from build123d import *

# Parameters (mm, degrees)
SKIZZE1_W                       = 22
SKIZZE1_H                       = 72.8
AUFSATZ_LINEAR_AUSTRAGEN1_DEPTH = 2
SKIZZE2_R                       = 3
SCHNITT_LINEAR_AUSTRAGEN1_DEPTH = 2
SKIZZE3_W                       = 65.5
SKIZZE3_H                       = 21
AUFSATZ_LINEAR_AUSTRAGEN2_DEPTH = 2.8
SCHNITT_LINEAR_AUSTRAGEN2_DEPTH = 67.590464783
SKIZZE5_R                       = 3
SCHNITT_LINEAR_AUSTRAGEN4_DEPTH = 39.128729326
SKIZZE6_W                       = 18
SKIZZE6_H                       = 1
SCHNITT_LINEAR_AUSTRAGEN5_DEPTH = 40
SKIZZE8_W                       = 15
SKIZZE8_H                       = 10
SCHNITT_LINEAR_AUSTRAGEN6_DEPTH = 0.5
VERRUNDUNG3_R                   = 1
SKIZZE9_W                       = 5
SKIZZE9_H                       = 12
AUFSATZ_LINEAR_AUSTRAGEN3_DEPTH = 8
SKIZZE10_W                      = 10
SKIZZE10_H                      = 5
SCHNITT_LINEAR_AUSTRAGEN7_DEPTH = 75.236715983


with BuildPart() as part:
    # Skizze1 → Aufsatz-Linear austragen1 (new body)
    with BuildSketch(Plane(origin=(0, 0, 0), x_dir=(0, 1, 0), z_dir=(0, 0, 1))):
        Rectangle(SKIZZE1_W, SKIZZE1_H)
    extrude(amount=AUFSATZ_LINEAR_AUSTRAGEN1_DEPTH)

    # Skizze2 → Schnitt-Linear austragen1 (cut)
    with BuildSketch(Plane.XY.offset(2)):
        with Locations((-34.28, 8.88)):
            Circle(SKIZZE2_R)
        with Locations((-34.28, -8.88)):
            Circle(SKIZZE2_R)
        with Locations((34.28, -8.88)):
            Circle(SKIZZE2_R)
        with Locations((34.28, 8.88)):
            Circle(SKIZZE2_R)
    extrude(amount=-SCHNITT_LINEAR_AUSTRAGEN1_DEPTH, mode=Mode.SUBTRACT)

    # Skizze3 → Aufsatz-Linear austragen2 (add)
    with BuildSketch(Plane.XY.offset(2)):
        with Locations((3.65, 0)):
            Rectangle(SKIZZE3_W, SKIZZE3_H)
    extrude(amount=AUFSATZ_LINEAR_AUSTRAGEN2_DEPTH)

    # Skizze4 → Schnitt-Linear austragen2 (cut, through all)
    with BuildSketch(Plane(origin=(-29.1, 0, 0), x_dir=(0, -1, 0), z_dir=(-1, 0, 0))):
        Polygon((-8, 4.8), (8, 4.8), (8, 4.1), (9, 4.1), (9, 2), (-9, 2), (-9, 4.1), (-8, 4.1), align=None)
    extrude(amount=-SCHNITT_LINEAR_AUSTRAGEN2_DEPTH, mode=Mode.SUBTRACT)

    # Skizze5 → Schnitt-Linear austragen4 (cut, through all)
    with BuildSketch(Plane(origin=(0, 0, 2), x_dir=(1, 0, 0), z_dir=(0, 0, -1))):
        with Locations((34.28, -8.88)):
            Circle(SKIZZE5_R)
        with Locations((34.28, 8.88)):
            Circle(SKIZZE5_R)
    extrude(amount=-SCHNITT_LINEAR_AUSTRAGEN4_DEPTH, mode=Mode.SUBTRACT)

    # Skizze6 → Schnitt-Linear austragen5 (cut)
    with BuildSketch(Plane(origin=(-36.4, 0, 0), x_dir=(0, -1, 0), z_dir=(-1, 0, 0))):
        with Locations((0, 2)):
            Rectangle(SKIZZE6_W, SKIZZE6_H)
    extrude(amount=-SCHNITT_LINEAR_AUSTRAGEN5_DEPTH, mode=Mode.SUBTRACT)

    # Skizze8 → Schnitt-Linear austragen6 (cut)
    with BuildSketch(Plane.XY.offset(2)):
        with Locations((8.655984658, -0.007335612)):
            Rectangle(SKIZZE8_W, SKIZZE8_H)
    extrude(amount=-SCHNITT_LINEAR_AUSTRAGEN6_DEPTH, mode=Mode.SUBTRACT)

    # Verrundung3
    # the kernel refuses this fillet: 1 mm, written as the material it adds along each edge
    with BuildSketch(Plane(origin=(3.6, -9, 1.5), x_dir=(0, 0, 1), z_dir=(0, 1, 0))) as verrundung3_piece_1:
        with BuildLine():
            CenterArc((1, -0.866025404), VERRUNDUNG3_R, 120, 60)
            Line((0, -0.866025404), (-0.02, -0.866025404))
            Line((-0.02, -0.866025404), (-0.02, 0))
            Line((-0.02, 0), (0, 0.02))
            ThreePointArc((0, 0.02), (0.25, 0.02), (0.49, 0.017320508))
            Line((0.49, 0.017320508), (0.5, 0))
        make_face()
    extrude(amount=3.992664388)
    with BuildSketch(Plane(origin=(3.6, -5.007335612, 1.5), x_dir=(0, 0, 1), z_dir=(1, 0, 0)), Plane(origin=(16.155984658, 4.992664388, 1.5), x_dir=(0, 0, 1), z_dir=(-1, 0, 0))) as verrundung3_piece_2:
        with BuildLine():
            CenterArc((1, -0.866025404), VERRUNDUNG3_R, 120, 60)
            Line((0, -0.866025404), (-0.02, -0.866025404))
            Line((-0.02, -0.866025404), (-0.02, 0))
            Line((-0.02, 0), (0, 0.02))
            ThreePointArc((0, 0.02), (0.25, 0.02), (0.49, 0.017320508))
            Line((0.49, 0.017320508), (0.5, 0))
        make_face()
    extrude(amount=12.555984658)
    with BuildSketch(Plane(origin=(3.6, 4.992664388, 1.5), x_dir=(0, 0, 1), z_dir=(0, 1, 0))) as verrundung3_piece_3:
        with BuildLine():
            CenterArc((1, -0.866025404), VERRUNDUNG3_R, 120, 60)
            Line((0, -0.866025404), (-0.02, -0.866025404))
            Line((-0.02, -0.866025404), (-0.02, 0))
            Line((-0.02, 0), (0, 0.02))
            ThreePointArc((0, 0.02), (0.25, 0.02), (0.49, 0.017320508))
            Line((0.49, 0.017320508), (0.5, 0))
        make_face()
    extrude(amount=4.007335612)
    with BuildSketch(Plane(origin=(16.155984658, -5.007335612, 1.5), x_dir=(0, 0, 1), z_dir=(0, 1, 0))) as verrundung3_piece_4:
        with BuildLine():
            CenterArc((1, -0.866025404), VERRUNDUNG3_R, 120, 60)
            Line((0, -0.866025404), (-0.02, -0.866025404))
            Line((-0.02, -0.866025404), (-0.02, 0))
            Line((-0.02, 0), (0, 0.02))
            ThreePointArc((0, 0.02), (0.25, 0.02), (0.49, 0.017320508))
            Line((0.49, 0.017320508), (0.5, 0))
        make_face()
    extrude(amount=10)
    with BuildSketch(Plane(origin=(3.6, -9, 1.5), x_dir=(0, 0, 1), z_dir=(0, 1, 0))) as verrundung3_piece_5a_section:
        with BuildLine():
            CenterArc((1, -0.866025404), VERRUNDUNG3_R, 120, 60)
            Line((0, -0.866025404), (-0.02, -0.866025404))
            Line((-0.02, -0.866025404), (-0.02, 0))
            Line((-0.02, 0), (0, 0.02))
            ThreePointArc((0, 0.02), (0.25, 0.02), (0.49, 0.017320508))
            Line((0.49, 0.017320508), (0.5, 0))
        make_face()
    verrundung3_piece_5a = extrude(amount=6.157727897, mode=Mode.PRIVATE)
    verrundung3_piece_5a = split(verrundung3_piece_5a, bisect_by=Plane(origin=(3.383689554, -5.007335612, 1.629516711), z_dir=(0, 1, 0)), keep=Keep.TOP, mode=Mode.PRIVATE)
    with BuildSketch(Plane(origin=(1.434936491, -5.007335612, 1.5), x_dir=(0, 0, 1), z_dir=(1, 0, 0))) as verrundung3_piece_5b_section:
        with BuildLine():
            CenterArc((1, -0.866025404), VERRUNDUNG3_R, 120, 60)
            Line((0, -0.866025404), (-0.02, -0.866025404))
            Line((-0.02, -0.866025404), (-0.02, 0))
            Line((-0.02, 0), (0, 0.02))
            ThreePointArc((0, 0.02), (0.25, 0.02), (0.49, 0.017320508))
            Line((0.49, 0.017320508), (0.5, 0))
        make_face()
    verrundung3_piece_5b = extrude(amount=14.721048168, mode=Mode.PRIVATE)
    verrundung3_piece_5b = split(verrundung3_piece_5b, bisect_by=Plane(origin=(3.6, -4.791025166, 1.629516711), z_dir=(-1, 0, 0)), keep=Keep.TOP, mode=Mode.PRIVATE)
    verrundung3_piece_5 = verrundung3_piece_5a & verrundung3_piece_5b
    add(verrundung3_piece_5)
    with BuildSketch(Plane(origin=(3.6, -5.007335612, 1.5), x_dir=(0, 0, 1), z_dir=(1, 0, 0))) as verrundung3_piece_6a_section:
        with BuildLine():
            CenterArc((1, -0.866025404), VERRUNDUNG3_R, 120, 60)
            Line((0, -0.866025404), (-0.02, -0.866025404))
            Line((-0.02, -0.866025404), (-0.02, 0))
            Line((-0.02, 0), (0, 0.02))
            ThreePointArc((0, 0.02), (0.25, 0.02), (0.49, 0.017320508))
            Line((0.49, 0.017320508), (0.5, 0))
        make_face()
    verrundung3_piece_6a = extrude(amount=14.721048168, mode=Mode.PRIVATE)
    verrundung3_piece_6a = split(verrundung3_piece_6a, bisect_by=Plane(origin=(16.155984658, -4.791025166, 1.629516711), z_dir=(1, 0, 0)), keep=Keep.TOP, mode=Mode.PRIVATE)
    with BuildSketch(Plane(origin=(16.155984658, -7.172399122, 1.5), x_dir=(0, 0, 1), z_dir=(0, 1, 0))) as verrundung3_piece_6b_section:
        with BuildLine():
            CenterArc((1, -0.866025404), VERRUNDUNG3_R, 120, 60)
            Line((0, -0.866025404), (-0.02, -0.866025404))
            Line((-0.02, -0.866025404), (-0.02, 0))
            Line((-0.02, 0), (0, 0.02))
            ThreePointArc((0, 0.02), (0.25, 0.02), (0.49, 0.017320508))
            Line((0.49, 0.017320508), (0.5, 0))
        make_face()
    verrundung3_piece_6b = extrude(amount=12.165063509, mode=Mode.PRIVATE)
    verrundung3_piece_6b = split(verrundung3_piece_6b, bisect_by=Plane(origin=(15.939674213, -5.007335612, 1.629516711), z_dir=(0, -1, 0)), keep=Keep.TOP, mode=Mode.PRIVATE)
    verrundung3_piece_6 = verrundung3_piece_6a & verrundung3_piece_6b
    add(verrundung3_piece_6)
    with BuildSketch(Plane(origin=(16.155984658, 4.992664388, 1.5), x_dir=(0, 0, 1), z_dir=(-1, 0, 0))) as verrundung3_piece_7a_section:
        with BuildLine():
            CenterArc((1, -0.866025404), VERRUNDUNG3_R, 120, 60)
            Line((0, -0.866025404), (-0.02, -0.866025404))
            Line((-0.02, -0.866025404), (-0.02, 0))
            Line((-0.02, 0), (0, 0.02))
            ThreePointArc((0, 0.02), (0.25, 0.02), (0.49, 0.017320508))
            Line((0.49, 0.017320508), (0.5, 0))
        make_face()
    verrundung3_piece_7a = extrude(amount=14.721048168, mode=Mode.PRIVATE)
    verrundung3_piece_7a = split(verrundung3_piece_7a, bisect_by=Plane(origin=(3.6, 4.776353942, 1.629516711), z_dir=(-1, 0, 0)), keep=Keep.TOP, mode=Mode.PRIVATE)
    with BuildSketch(Plane(origin=(3.6, 2.827600878, 1.5), x_dir=(0, 0, 1), z_dir=(0, 1, 0))) as verrundung3_piece_7b_section:
        with BuildLine():
            CenterArc((1, -0.866025404), VERRUNDUNG3_R, 120, 60)
            Line((0, -0.866025404), (-0.02, -0.866025404))
            Line((-0.02, -0.866025404), (-0.02, 0))
            Line((-0.02, 0), (0, 0.02))
            ThreePointArc((0, 0.02), (0.25, 0.02), (0.49, 0.017320508))
            Line((0.49, 0.017320508), (0.5, 0))
        make_face()
    verrundung3_piece_7b = extrude(amount=6.172399122, mode=Mode.PRIVATE)
    verrundung3_piece_7b = split(verrundung3_piece_7b, bisect_by=Plane(origin=(3.383689554, 4.992664388, 1.629516711), z_dir=(0, -1, 0)), keep=Keep.TOP, mode=Mode.PRIVATE)
    verrundung3_piece_7 = verrundung3_piece_7a & verrundung3_piece_7b
    add(verrundung3_piece_7)
    with BuildSketch(Plane(origin=(16.155984658, -5.007335612, 1.5), x_dir=(0, 0, 1), z_dir=(0, 1, 0))) as verrundung3_piece_8a_section:
        with BuildLine():
            CenterArc((1, -0.866025404), VERRUNDUNG3_R, 120, 60)
            Line((0, -0.866025404), (-0.02, -0.866025404))
            Line((-0.02, -0.866025404), (-0.02, 0))
            Line((-0.02, 0), (0, 0.02))
            ThreePointArc((0, 0.02), (0.25, 0.02), (0.49, 0.017320508))
            Line((0.49, 0.017320508), (0.5, 0))
        make_face()
    verrundung3_piece_8a = extrude(amount=12.165063509, mode=Mode.PRIVATE)
    verrundung3_piece_8a = split(verrundung3_piece_8a, bisect_by=Plane(origin=(15.939674213, 4.992664388, 1.629516711), z_dir=(0, 1, 0)), keep=Keep.TOP, mode=Mode.PRIVATE)
    with BuildSketch(Plane(origin=(18.321048168, 4.992664388, 1.5), x_dir=(0, 0, 1), z_dir=(-1, 0, 0))) as verrundung3_piece_8b_section:
        with BuildLine():
            CenterArc((1, -0.866025404), VERRUNDUNG3_R, 120, 60)
            Line((0, -0.866025404), (-0.02, -0.866025404))
            Line((-0.02, -0.866025404), (-0.02, 0))
            Line((-0.02, 0), (0, 0.02))
            ThreePointArc((0, 0.02), (0.25, 0.02), (0.49, 0.017320508))
            Line((0.49, 0.017320508), (0.5, 0))
        make_face()
    verrundung3_piece_8b = extrude(amount=14.721048168, mode=Mode.PRIVATE)
    verrundung3_piece_8b = split(verrundung3_piece_8b, bisect_by=Plane(origin=(16.155984658, 4.776353942, 1.629516711), z_dir=(1, 0, 0)), keep=Keep.TOP, mode=Mode.PRIVATE)
    verrundung3_piece_8 = verrundung3_piece_8a & verrundung3_piece_8b
    add(verrundung3_piece_8)

    # Skizze9 → Aufsatz-Linear austragen3 (add)
    with BuildSketch(Plane.XY.offset(1.5)):
        with Locations((-33.9, 0)):
            Rectangle(SKIZZE9_W, SKIZZE9_H)
    extrude(amount=AUFSATZ_LINEAR_AUSTRAGEN3_DEPTH)

    # Skizze10 → Schnitt-Linear austragen7 (cut, through all)
    with BuildSketch(Plane(origin=(-36.4, 0, 0), x_dir=(0, -1, 0), z_dir=(-1, 0, 0))):
        with Locations((0, 5.5)):
            Rectangle(SKIZZE10_W, SKIZZE10_H)
    extrude(amount=-SCHNITT_LINEAR_AUSTRAGEN7_DEPTH, mode=Mode.SUBTRACT)


solid = part.part
Could you check a few things on this model? Use its own coordinates, in mm. A direction names the side the tool comes from. Coordinates: 2 decimals unless noted, no trailing zeros. Loops run counter-clockwise (first coordinate to the right, second up) from the corner with the lowest first, then second, coordinate; pieces in that order, holes last. Notation, with made-up numbers: (53, -33.5) -> (66, -33.5) arc R12 cw to (66, -15.5) -> close; hole circle Ø10 at (-11.5, 88.5). An arc over 180 degrees is marked (long way). Answer in a Markdown table with one row per item.
(1) If I drill on probe 1 along Y at (x, z) = (8, 4.5); probe 2 along X at (y, z) = (5.75, 3.5); probe 3 along Z at (x, y) = (-25.5, 8.25), over which ranges is the centre line in solid material (lowest first)?
Results found:
| item | result |
|---|---|
| probe 1 | y = -10.5 to -8, 8 to 10.5 |
| probe 2 | x = -36.4 to -31.4 |
| probe 3 | z = 0 to 1.5, 4.1 to 4.8 |
(2) Imagine slicing it at D-D (x = -6). List the corners of the cut face in (y, z) for me.
Results found:
| item | result |
|---|---|
| outline | (-11, 0) -> (11, 0) -> (11, 2) -> (10.5, 2) -> (10.5, 4.8) -> (8, 4.8) -> (8, 4.1) -> (9, 4.1) -> (9, 1.5) -> (-9, 1.5) -> (-9, 4.1) -> (-8, 4.1) -> (-8, 4.8) -> (-10.5, 4.8) -> (-10.5, 2) -> (-11, 2) -> close |
(3) Thinking about a two-plate mould opening in Z: for faces 5 (the face through (1, -10.5, 3)), 6 (the face through (-34, 0, 3)), 7 (the face through (1, -9, 4.8)), which applies, released by +Z, released by -Z, zero draft, split by the parting line, or undercut?
Results found:
| item | result |
|---|---|
| face 5 | zero draft |
| face 6 | undercut |
| face 7 | released by +Z |
(4) Will these pins go through, and if not, where does the flat tip stop? pin 1 Ø0.8 at (x, z) = (9.5, 4.5) entering from +Y; pin 2 Ø6 at (x, y) = (14.5, -4.5) entering from +Z; pin 3 Ø2 at (x, z) = (11.5, 4) entering from -Y; pin 4 Ø1 at (y, z) = (0, 6) entering from -X.
Results found:
| item | result |
|---|---|
| pin 1 | stops at y = 10.5 |
| pin 2 | stops at z = 2 |
| pin 3 | stops at y = -10.5 |
| pin 4 | passes through |
(5) Imagine slicing it at B-B (y = 1.25). List the corners of the cut face in (x, z) for me.
Results found:
| item | result |
|---|---|
| outline | (-36.4, 0) -> (36.4, 0) -> (36.4, 2) -> (16.16, 2) arc R1 cw to (15.29, 1.5) -> (-31.4, 1.5) -> (-31.4, 3) -> (-36.4, 3) -> close; (-36.4, 8) -> (-31.4, 8) -> (-31.4, 9.5) -> (-36.4, 9.5) -> close |
(6) Imagine slicing it at C-C (z = 5.5). List the corners of the cut face in (x, y) for me.
Results found:
| item | result |
|---|---|
| outline | (-36.4, -6) -> (-31.4, -6) -> (-31.4, -5) -> (-36.4, -5) -> close; (-36.4, 5) -> (-31.4, 5) -> (-31.4, 6) -> (-36.4, 6) -> close |
(7) For faces 1 (the face through (-34, 0, 8)), 2 (the face through (1, 10.5, 3)), 3 (the face through (-32.11, -6.81, 0.79)), 4 (the face through (-29.1, 10, 4)), which set-ups out of +Z, -Z, +X, -X, +Y, -Y let a thin tool reach every point of the face, with its end or its side?
Results found:
| item | result |
|---|---|
| face 1 | +X, -X |
| face 2 | +Z, +X, -X, +Y |
| face 3 | -Z |
| face 4 | +Z, -X, +Y, -Y |
(8) Imagine slicing it at A-A (x = -34.28). List the corners of the cut face in (y, z) for me, plus the area to 3 significant figures.
Results found:
| item | result |
|---|---|
| outline | (-6, 1.5) -> (-5.88, 1.5) -> (-5.88, 0) -> (5.88, 0) -> (5.88, 1.5) -> (6, 1.5) -> (6, 9.5) -> (-6, 9.5) -> close; hole (-5, 3) -> (5, 3) -> (5, 8) -> (-5, 8) -> close |
| area | 63.6 mm^2 |
